Geometry: final body of the model. Coordinates: model frame, mm. A direction names the side the tool comes from. Give positions to 0.01 mm unless a question says otherwise; leave off trailing zeros. Loops run counter-clockwise (first coordinate to the right, second up) from the corner with the lowest first, then second, coordinate; pieces in that order, holes last.
1. Section B-B, the plane x = 0. Output: boundary loops of the cut face in (y, z) (3 decimals), then the cut area to 3 significant figures.
2. Access query for faces 1 (the face through (0, -12.446, 3)), 2 (the face through (-2, -8, 12)), 3 (the face through (0, -6, 2.535)), 4 (the face through (-0.44, -10.16, -7.41)). Directions: +Z, -Z, +X, -X, +Y, -Y. A direction counts if a zero-diameter tool reaches every point of the face in a straight line with its end or side. Return the directions, or none.
3. First-contact query: P1, Ø5, axis at x = 0.5, y = -8, coming from the +Z side; P2, Ø4, axis at x = 22, z = 20, coming from the -Y side; P3, Ø3, axis at x = -20.5, y = -2.5, coming from the +Z side. Flat tips, straight axial feed; report the tip coordinate or a pass-through.
4. Material intervals for line 1 along Z through (x, y) = (0, -2.25) (3 decimals); line 2 along Z through (x, y) = (15.5, -3.75); line 3 along Y through (x, z) = (-12.5, 25), sorted ascending.
5. Draft query along X for faces 5 (the face through (-5.623, -6.136, -0.177)), 6 (the face through (0, 0, -6)), 7 (the face through (-28.547, -1.941, 1.256)). Return one class per face: +X half, -X half, draft (parallel to the pull), parting line (faces both ways), or undercut.
6. Section A-A, the plane z = 0. Output: boundary loops of the cut face in (x, y) (3 decimals).
7. Section C-C, the plane y = -2.5. State how many separate pieces and enclosed holes the cut face has, then the cut area to 3 significant figures.
8. Section D-D, the plane z = -17.5. Output: boundary loops of the cut face in (x, y).
from build123d import *

# Parameters (mm, degrees)
F0_R     = 12.1666
F1_DEPTH = 12.446
F0_R_2   = 28.575
F0_R_3   = 2.5908
F0_R_4   = 2.506168
F2_DEPTH = 3.937
F3_R     = 2.0193
F4_DEPTH = 25.4


with BuildPart() as f1:
    # F0 (on Front) → F1 (new body)
    with BuildSketch(Plane.XZ):
        Circle(F0_R)
        with BuildLine():
            ThreePointArc((-4.892358, -2.778407), (-5.624556, -0.138136), (-5.02285, 2.534895))
            Line((-5.02285, 2.534895), (5.02285, 2.534895))
            ThreePointArc((5.02285, 2.534895), (5.624556, -0.138136), (4.892358, -2.778407))
            Line((4.892358, -2.778407), (-4.892358, -2.778407))
        make_face(mode=Mode.SUBTRACT)
    extrude(amount=F1_DEPTH)

    # F0 (on Front) → F2 (join)
    with BuildSketch(Plane.XZ):
        Circle(F0_R_2)
        with Locations((-17.251513, -16.192724)):
            Circle(F0_R_3, mode=Mode.SUBTRACT)
        with Locations((0, -23.660495)):
            Circle(F0_R_3, mode=Mode.SUBTRACT)
        with Locations((17.595791, -15.817938)):
            Circle(F0_R_3, mode=Mode.SUBTRACT)
        with Locations((-23.660495, 0)):
            Circle(F0_R_4, mode=Mode.SUBTRACT)
        with Locations((-15.588157, 17.799674)):
            Circle(F0_R_3, mode=Mode.SUBTRACT)
        Circle(F0_R, mode=Mode.SUBTRACT)
        with Locations((23.660495, 0)):
            Circle(F0_R_3, mode=Mode.SUBTRACT)
        with Locations((0, 23.660495)):
            Circle(F0_R_3, mode=Mode.SUBTRACT)
        with Locations((16.086078, 17.350997)):
            Circle(F0_R_3, mode=Mode.SUBTRACT)
    extrude(amount=F2_DEPTH)

    # F3 (on Top) → F4 (cut)
    with BuildSketch(Plane.XY):
        with Locations((0, -8.190851)):
            Circle(F3_R)
    extrude(amount=-F4_DEPTH, mode=Mode.SUBTRACT)


solid = f1.part
Answers below:
1. outline: (-12.446, -12.167) - (-10.21, -12.167) - (-10.21, -2.778) - (-12.446, -2.778) - close; (-12.446, 2.535) - (0, 2.535) - (0, 21.07) - (-3.937, 21.07) - (-3.937, 12.167) - (-12.446, 12.167) - close; (-6.172, -12.167) - (-3.937, -12.167) - (-3.937, -21.07) - (0, -21.07) - (0, -2.778) - (-6.172, -2.778) - close; (-3.937, -28.575) - (0, -28.575) - (0, -26.251) - (-3.937, -26.251) - close; (-3.937, 26.251) - (0, 26.251) - (0, 28.575) - (-3.937, 28.575) - close
1. area: 287 mm2
2. face 1: +Z, -Z, +X, -X, -Y
2. face 2: -Y
2. face 3: +Y, -Y
2. face 4: -Z
3. P1: stops at z = 12.17
3. P2: stops at y = -3.94
3. P3: stops at z = 21.34
4. line 1: z = -28.575 to -26.251, -21.07 to -2.778, 2.535 to 21.07, 26.251 to 28.575
4. line 2: z = -24.01 to -17.34, -14.29 to 14.83, 19.87 to 24.01
4. line 3: y = -3.94 to 0
5. face 5: undercut
5. face 6: draft
5. face 7: parting line
6. outline: (-28.575, -3.937) - (-26.167, -3.937) - (-26.167, 0) - (-28.575, 0) - close; (-21.154, -3.937) - (-12.167, -3.937) - (-12.167, -12.446) - (-5.626, -12.446) - (-5.626, 0) - (-21.154, 0) - close; (5.626, -12.446) - (12.167, -12.446) - (12.167, -3.937) - (21.07, -3.937) - (21.07, 0) - (5.626, 0) - close; (26.251, -3.937) - (28.575, -3.937) - (28.575, 0) - (26.251, 0) - close
7. separate pieces: 1
7. enclosed holes: 9
7. area: 2,340 mm2
8. outline: (-22.59, -3.94) - (-19.49, -3.94) - (-19.49, 0) - (-22.59, 0) - close; (-15.01, -3.94) - (15.63, -3.94) - (15.63, 0) - (-15.01, 0) - close; (19.57, -3.94) - (22.59, -3.94) - (22.59, 0) - (19.57, 0) - close
